```python
from build123d import *

# Parameters (mm, degrees)
F0_W     = 105.438776
F0_H     = 85.334472
F1_DEPTH = 25.4
F2_R     = 15.310247
F3_DEPTH = 25.4
F5_DEPTH = 87.376


with BuildPart() as f1:
    # F0 (on Top) → F1 (new body)
    with BuildSketch(Plane.XY):
        Rectangle(F0_W, F0_H)
    extrude(amount=F1_DEPTH)

    # F2 (on face) → F3 (join)
    with BuildSketch(Plane.XY.offset(25.4)):
        Circle(F2_R)
    extrude(amount=F3_DEPTH)

    # F4 (on face) → F5 (cut)
    with BuildSketch(Plane(origin=(0, 42.667236, 0), x_dir=(-1, 0, 0), z_dir=(0, 1, 0))):
        Polygon((-27.478183, 63.615456), (-29.094545, 48.837271), (23.552727, 31.750001), (32.437156, 59.123653), align=None)
    extrude(amount=-F5_DEPTH, mode=Mode.SUBTRACT)


solid = f1.part
```
Could you check a few things on this model? Use its own coordinates, in mm. A direction names the side the tool comes from. Coordinates: 2 decimals unless noted, no trailing zeros. Write each loop counter-clockwise with the first axis right and the second up, starting at its lowest first coordinate (ties: lowest second). Pieces come first, ordered by that corner, then holes. Notation, with made-up numbers: (-14.75, 42) - (22.25, 42) arc R35 ccw to (22.25, 81) - close; hole circle Ø4 at (41.5, 81.25). An arc over 180 degrees is marked (long way). Use a Markdown table: item, result.
Q1. Which directions (+Z, -Z, +X, -X, +Y, -Y) give clear straight access to the entire face, cutting with the end or side of a thin tool? Please do faces 1 (the flat face through (-52.719, -1, 13)), 2 (the cylindrical face through (14.603, 4.599, 32.642)).
Geometry check:
| item | result |
|---|---|
| face 1 | +Z, -Z, -X, +Y, -Y |
| face 2 | +Z |
Q2. I'm going to push flat-ended pins straight in: pin 1 Ø8 at (y, z) = (-26.5, 27) entering from -X; pin 2 Ø1.5 at (x, y) = (-23.5, -27.5) entering from +Z. Where does each tip first touch, or does it pass through?
Geometry check:
| item | result |
|---|---|
| pin 1 | stops at x = -52.72 |
| pin 2 | stops at z = 25.4 |
Q3. Imagine slicing it at C-C (z = 27). List the corners of the cut face in (x, y) for me.
Geometry check:
| item | result |
|---|---|
| outline | circle Ø30.62 at (0, 0) |
Q4. Imagine slicing it at D-D (x = -43.5). List the corners of the cut face in (y, z) for me.
Geometry check:
| item | result |
|---|---|
| outline | (-42.67, 0) - (42.67, 0) - (42.67, 25.4) - (-42.67, 25.4) - close |
Q5. Please list where these lines run through material, in increasing order: L1, parallel to Z at x = 18, y = -13; L2, parallel to Y at x = 4.5, z = 33; L3, parallel to Z at x = 1.5, y = 6.
Geometry check:
| item | result |
|---|---|
| L1 | z = 0 to 25.4 |
| L2 | y = -14.63 to 14.63 |
| L3 | z = 0 to 39.88 |
Q6. Imagine slicing it at A-A (x = -3.5). List the corners of the cut face in (y, z) for me, and give its area (3 significant figures).
Geometry check:
| item | result |
|---|---|
| outline | (-42.67, 0) - (42.67, 0) - (42.67, 25.4) - (14.9, 25.4) - (14.9, 38.26) - (-14.9, 38.26) - (-14.9, 25.4) - (-42.67, 25.4) - close |
| area | 2,550 mm2 |
Q7. Thinking about a two-plate mould opening in Z: for faces 3 (the flat face through (-1, 42.667, 13)), 4 (the flat face through (-12, 10, 25.4)), 5 (the flat face through (-1, 1, 0)), which applies, +Z half, -Z half, draft (parallel to the pull), parting line (faces both ways), or undercut?
Geometry check:
| item | result |
|---|---|
| face 3 | draft |
| face 4 | +Z half |
| face 5 | -Z half |
Q8. Imagine slicing it at B-B (y = 0). List the corners of the cut face in (x, z) for me.
Geometry check:
| item | result |
|---|---|
| outline | (-52.72, 0) - (52.72, 0) - (52.72, 25.4) - (15.31, 25.4) - (15.31, 44.36) - (-15.31, 34.43) - (-15.31, 25.4) - (-52.72, 25.4) - close |
